Input: dimensioned drawing with shaded views. Units: mm. Origin: part minimum x, y, z. A direction names the side the tool comes from. Round coordinates to 2 decimals unless told otherwise and drop trailing zeros. Loops run counter-clockwise (first coordinate to the right, second up) from the corner with the lowest first, then second, coordinate; pieces in that order, holes last. Notation, with made-up numbers: (27.5, 4.5) - (83.5, 4.5) arc R20 ccw to (83.5, 13.5) - close; hole circle Ø9 at (33.25, -31.75). An arc over 180 degrees is marked (long way). One line per question, with ' | ' between items. Start each with the question number.
Item 1: First-contact query: pin 1 (2 mm diameter, centred on y = 28, z = 52, fed in from -X); pin 2 (8 mm diameter, centred on x = 23, z = 58.5, fed in from +Y); pin 3 (1.5 mm diameter, centred on y = 20, z = 139, fed in from +X). Flat tips, straight axial feed; report the tip coordinate or a pass-through.
Item 2: Material intervals for line 1 along Y through (x, z) = (24, 172); line 2 along Z through (x, y) = (33, 24); line 3 along X through (y, z) = (20.5, 133), sorted ascending.
Item 3: Section C-C, the plane z = 179.5. Return loops of the section in (x, y).
Item 4: Section A-A, the plane x = 22. Return loops of the section in (y, z) (3 decimals), plus the area to 3 significant figures.
Item 5: Set-up query: the marked faces 1 and 2. Return all of +Z, -Z, +X, -X, +Y, -Y with unobstructed straight access to the full face (end or side cutting, diameter ignored); none if empty.
Item 6: Section B-B, the plane y = 19.05. Return loops of the section in (x, z).
Item 7: Section D-D, the plane y = 10. Return loops of the section in (x, z), plus the area to 3 significant figures.
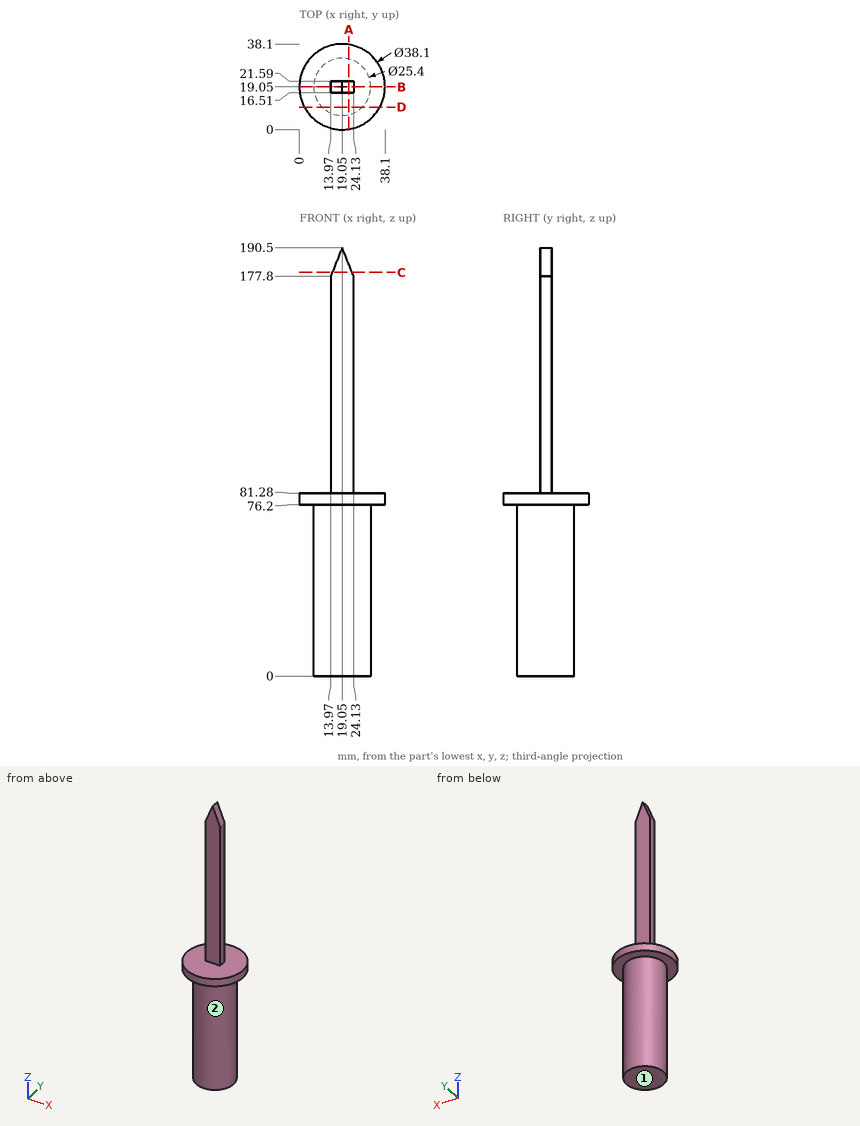
Return value:
1) pin 1: x = 9.15 | pin 2: y = 31.75 | pin 3: x = 24.13
2) line 1: 16.51 to 21.59 | line 2: 76.2 to 81.28 | line 3: 13.97 to 24.13
3) outline: (14.65, 16.51) - (23.45, 16.51) - (23.45, 21.59) - (14.65, 21.59) - close
4) outline: (0.23, 76.2) - (6.697, 76.2) - (6.697, 0) - (31.403, 0) - (31.403, 76.2) - (37.87, 76.2) - (37.87, 81.28) - (21.59, 81.28) - (21.59, 183.125) - (16.51, 183.125) - (16.51, 81.28) - (0.23, 81.28) - close | area: 2,590 mm2
5) face 1: -Z, +X, -X, +Y, -Y | face 2: -Z
6) outline: (0, 76.2) - (6.35, 76.2) - (6.35, 0) - (31.75, 0) - (31.75, 76.2) - (38.1, 76.2) - (38.1, 81.28) - (24.13, 81.28) - (24.13, 177.8) - (19.05, 190.5) - (13.97, 177.8) - (13.97, 81.28) - (0, 81.28) - close
7) outline: (2.29, 76.2) - (10.14, 76.2) - (10.14, 0) - (27.96, 0) - (27.96, 76.2) - (35.81, 76.2) - (35.81, 81.28) - (2.29, 81.28) - close | area: 1,530 mm2
